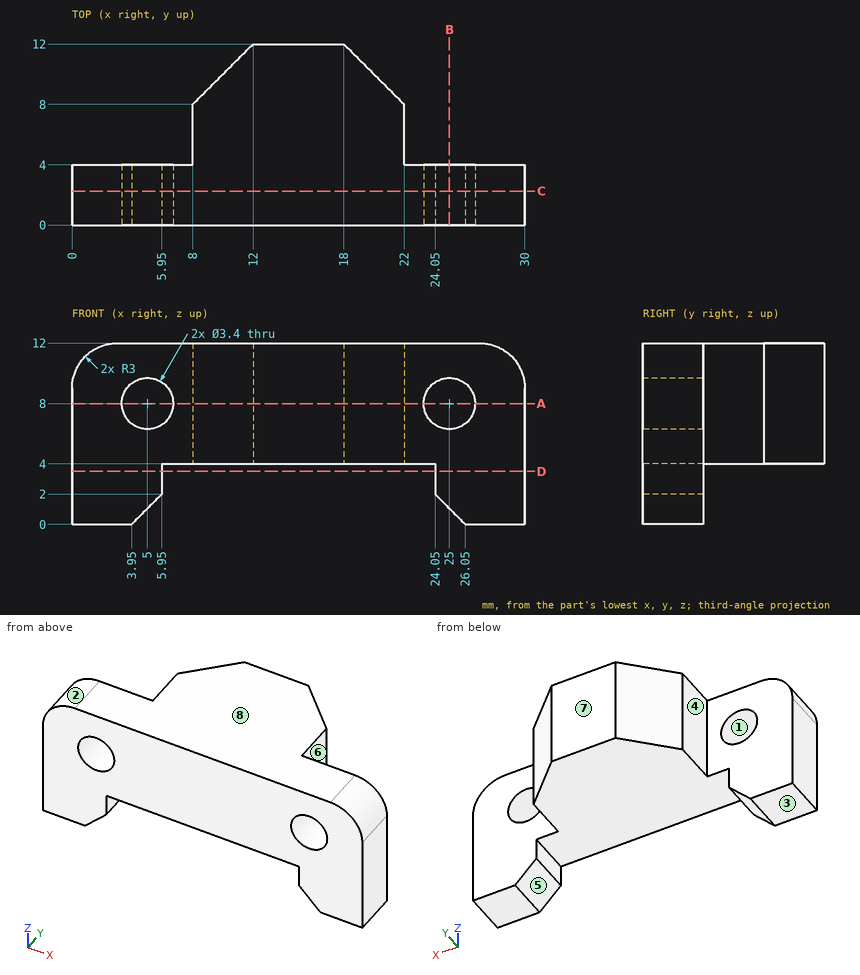
Study the drawing (mm; zero at the part's minimum x, y, z) and answer. A direction names the side the tool comes from. Round coordinates to 2 decimals unless told otherwise and drop trailing zeros. Loops run counter-clockwise (first coordinate to the right, second up) from the corner with the lowest first, then second, coordinate; pieces in that order, holes last.
Q1. Find the intervals of material crossed by line 1 (X direction, y = 1.9, z = 8); line 2 (Z direction, x = 21, y = 8.5); line 3 (Y direction, x = 21, z = 6), in increasing order.
Q2. Section A-A, the plane z = 8 is taken. Determine the outline of the cut face in (x, y).
Q3. For a pull along Z with two mould halves and no side action, classify the marked faces 1, 2 and 3 as released by +Z, released by -Z, zero draft, split by the parting line, or undercut.
Q4. Section B-B, the plane x = 25 is taken. Determine the outline of the cut face in (y, z), then the cut area to 3 significant figures.
Q5. Section C-C, the plane y = 2.25 is taken. Determine the outline of the cut face in (x, z).
Q6. Given pin 1 Ø4 at (x, z) = (24.5, 5) entering from +Y; pin 2 Ø3.5 at (x, y) = (16.5, 5.5) entering from -Z; pin 3 Ø4.5 at (y, z) = (6.5, 7.5) entering from -X, each flat-ended and moving along its own axis, determine where each tip first touches the part or whether it passes through.
Q7. Section D-D, the plane z = 3.5 is taken. Determine the outline of the cut face in (x, y).
Q8. Which of the six approach directions +Z, -Z, +X, -X, +Y, -Y give full straight-line access (tool end or side, diameter ignored) to the marked faces 4, 5, 6, 7 and 8?
Completed:
1. line 1: x = 0 to 3.3, 6.7 to 23.3, 26.7 to 30
1. line 2: z = 4 to 12
1. line 3: y = 0 to 9
2. outline: (0, 0) - (3.3, 0) - (3.3, 4) - (0, 4) - close; (6.7, 0) - (23.3, 0) - (23.3, 4) - (22, 4) - (22, 8) - (18, 12) - (12, 12) - (8, 8) - (8, 4) - (6.7, 4) - close; (26.7, 0) - (30, 0) - (30, 4) - (26.7, 4) - close
3. face 1: undercut
3. face 2: released by +Z
3. face 3: released by -Z
4. outline: (0, 1.05) - (4, 1.05) - (4, 6.3) - (0, 6.3) - close; (0, 9.7) - (4, 9.7) - (4, 12) - (0, 12) - close
4. area: 30.2 mm2
5. outline: (0, 0) - (3.95, 0) - (5.95, 2) - (5.95, 4) - (24.05, 4) - (24.05, 2) - (26.05, 0) - (30, 0) - (30, 9) arc R3 ccw to (27, 12) - (3, 12) arc R3 ccw to (0, 9) - close; hole circle Ø3.4 at (5, 8); hole circle Ø3.4 at (25, 8)
6. pin 1: stops at y = 4
6. pin 2: stops at z = 4
6. pin 3: stops at x = 8
7. outline: (0, 0) - (5.95, 0) - (5.95, 4) - (0, 4) - close; (24.05, 0) - (30, 0) - (30, 4) - (24.05, 4) - close
8. face 4: +Z, -Z, -X, +Y
8. face 5: -Z, +Y, -Y
8. face 6: +Z, -Z, +X, +Y
8. face 7: +Z, -Z, +X, -X, +Y
8. face 8: +Z, +X, -X, +Y, -Y
